The drawing under review shows one solid part. Ordinate dimensions are in mm from its lowest x, y, z. A direction names the side the tool comes from. Give positions to 0.01 mm unless a question says otherwise; leave off trailing zeros. Loops run counter-clockwise (first coordinate to the right, second up) from the corner with the lowest first, then second, coordinate; pieces in that order, holes last. Notation, with made-up numbers: M -19,-30 L 38,-30 A16 cw 38,-22 Z; hole C 24,9.5 d10. An arc over 180 degrees is marked long. One line per item, written item: value. Start each with the question number.
Q1. For the marked faces 1 and 2, list the 3-axis set-ups (+Z, -Z, +X, -X, +Y, -Y) from which the entire face can be reached by the end or side of a thin tool; tool diameter is ignored.
Q2. For pin 1 (3 mm diameter, centred on x = 6.5, y = 9, fed in from -Z); pin 2 (10 mm diameter, centred on x = 16.5, z = 42.5, fed in from +Y); pin 3 (7.5 mm diameter, centred on y = 9.525, z = 12.7, fed in from -X); pin 4 (4 mm diameter, centred on x = 11.5, z = 92, fed in from -Y), all flat-tipped, find the tip position at first contact; note any pin that passes through.
Q3. To check wall thickness, follow line 1 along Z through (x, y) = (11, 9); line 2 along X through (y, z) = (9.75, 157); line 3 along Y through (x, z) = (5.75, 12.7). State the ranges of each line that lie inside material, in increasing order. Write a range as from..to.
Q4. We need section B-B on z = 130.5. Write out the cut boundary in (x, y) (1 decimal), plus the area to 3 significant figures.
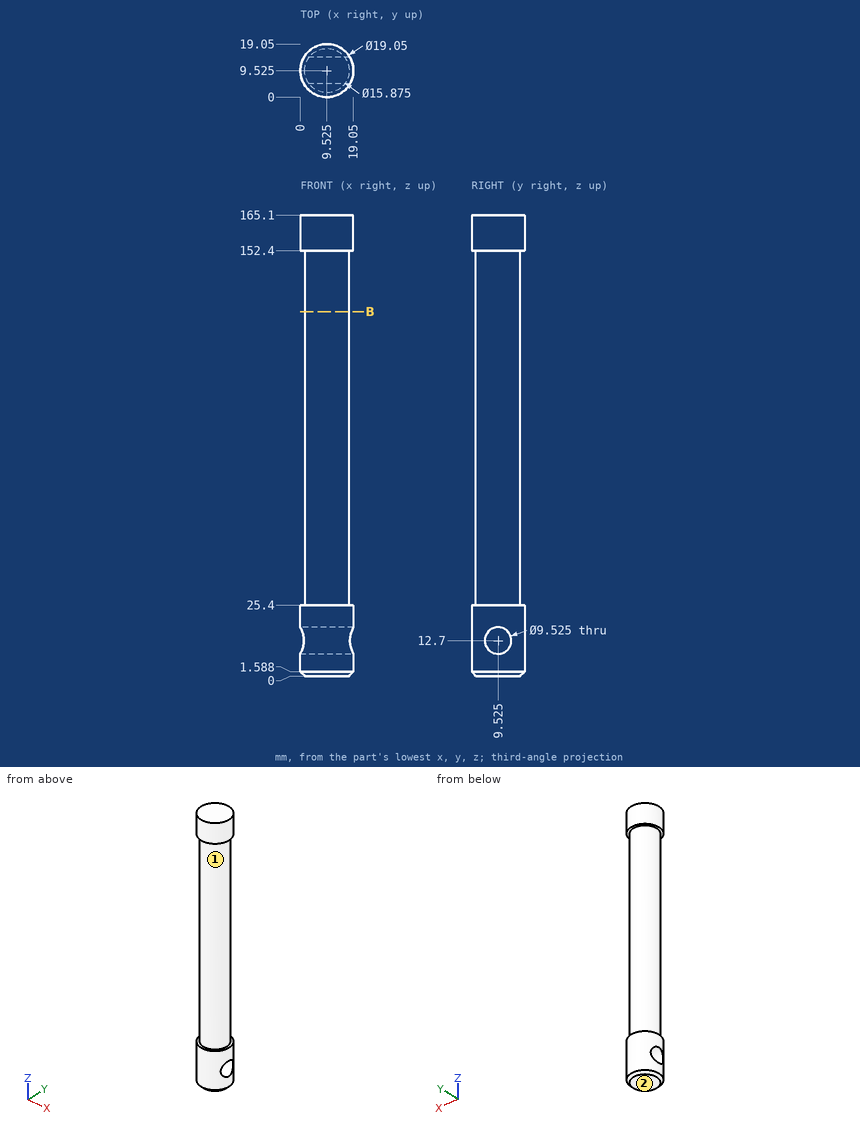
Solved:
1. face 1: none
1. face 2: -Z, +X, -X, +Y, -Y
2. pin 1: z = 0
2. pin 2: y = 17.21
2. pin 3: through
2. pin 4: y = 1.59
3. line 1: 0..7.97, 17.43..165.1
3. line 2: 0..19.05
3. line 3: 0.78..4.76, 14.29..18.27
4. outline: C 9.5,9.5 d15.9
4. area: 198 mm2
